from build123d import *

# Parameters (mm, degrees)
SKETCH_1_R      = 2.15
SKETCH_1_R_2    = 13.5
EXTRUDE_1_DEPTH = 5
FILLET_1_R      = 3
FILLET_2_R      = 1


with BuildPart() as part:
    # ｽｹｯﾁ1 → ﾎﾞｽ - 押し出し1 (new body)
    with BuildSketch(Plane(origin=(0, 0, 0), x_dir=(1, 0, 0), z_dir=(0, 1, 0))):
        with BuildLine():
            Line((-11.818899718, 2.076923077), (-16.328382426, -23.584655104))
            ThreePointArc((-16.328382426, -23.584655104), (-17.703637569, -26.24099819), (-20.349180229, -27.636917003))
            ThreePointArc((-20.349180229, -27.636917003), (-24.369978032, -31.689178902), (-21.971608059, -36.869474544))
            ThreePointArc((-21.971608059, -36.869474544), (-19.960473468, -39.083706455), (-19.573238085, -42.049770186))
            Line((-19.573238085, -42.049770186), (-20.683074506, -48.365384615))
            ThreePointArc((-20.683074506, -48.365384615), (-20.849535948, -54.509352655), (-19.230026487, -60.438369589))
            ThreePointArc((-19.230026487, -60.438369589), (-19.11671849, -64.1755701), (-21.627020352, -66.946470844))
            ThreePointArc((-21.627020352, -66.946470844), (-22.980970389, -74.980970389), (-14.946470844, -73.627020352))
            ThreePointArc((-14.946470844, -73.627020352), (-12.1755701, -71.11671849), (-8.438369589, -71.230026487))
            ThreePointArc((-8.438369589, -71.230026487), (-6.744432027, -71.887499507), (-5, -72.396078054))
            Line((-5, -72.396078054), (-5, -76.409830056))
            Line((-5, -76.409830056), (-2.666666667, -79.01857603))
            ThreePointArc((-2.666666667, -79.01857603), (3.651483717, -83.632993162), (-4, -82))
            Line((-4, -82), (-7.5, -82))
            ThreePointArc((-7.5, -82), (3.061862178, -88.846531969), (5, -76.409830056))
            Line((5, -76.409830056), (5, -72.396078054))
            ThreePointArc((5, -72.396078054), (6.744432027, -71.887499507), (8.438369589, -71.230026487))
            ThreePointArc((8.438369589, -71.230026487), (12.1755701, -71.11671849), (14.946470844, -73.627020352))
            ThreePointArc((14.946470844, -73.627020352), (22.980970389, -74.980970389), (21.627020352, -66.946470844))
            ThreePointArc((21.627020352, -66.946470844), (19.11671849, -64.1755701), (19.230026487, -60.438369589))
            ThreePointArc((19.230026487, -60.438369589), (20.849535948, -54.509352655), (20.683074506, -48.365384615))
            Line((20.683074506, -48.365384615), (19.573238085, -42.049770186))
            ThreePointArc((19.573238085, -42.049770186), (19.960473468, -39.083706455), (21.971608059, -36.869474544))
            ThreePointArc((21.971608059, -36.869474544), (24.369978032, -31.689178902), (20.349180229, -27.636917003))
            ThreePointArc((20.349180229, -27.636917003), (17.703637569, -26.24099819), (16.328382426, -23.584655104))
            Line((16.328382426, -23.584655104), (11.818899718, 2.076923077))
            ThreePointArc((11.818899718, 2.076923077), (0, 12), (-11.818899718, 2.076923077))
        make_face()
        with Locations(Location((-7.5, 0, 0), (0, 0, 270))):
            Circle(SKETCH_1_R, mode=Mode.SUBTRACT)
        with Locations(Location((7.5, 0, 0), (0, 0, 90))):
            Circle(SKETCH_1_R, mode=Mode.SUBTRACT)
        with Locations(Location((0, -52, 0), (0, 0, 270))):
            Circle(SKETCH_1_R_2, mode=Mode.SUBTRACT)
        with Locations(Location((19.445436483, -32.554563517, 0), (0, 0, 270))):
            Circle(SKETCH_1_R, mode=Mode.SUBTRACT)
        with Locations(Location((19.445436483, -71.445436483, 0), (0, 0, 270))):
            Circle(SKETCH_1_R, mode=Mode.SUBTRACT)
        with Locations(Location((-19.445436483, -71.445436483, 0), (0, 0, 270))):
            Circle(SKETCH_1_R, mode=Mode.SUBTRACT)
        with Locations(Location((-19.445436483, -32.554563517, 0), (0, 0, 270))):
            Circle(SKETCH_1_R, mode=Mode.SUBTRACT)
        with BuildLine():
            ThreePointArc((-4.384616486, -24.866395764), (0, -25.25), (4.384616486, -24.866395764))
            ThreePointArc((4.384616486, -24.866395764), (7.223675, -20.811800006), (3.169079242, -17.972741492))
            ThreePointArc((3.169079242, -17.972741492), (0, -18.25), (-3.169079242, -17.972741492))
            ThreePointArc((-3.169079242, -17.972741492), (-7.223675, -20.811800006), (-4.384616486, -24.866395764))
        make_face(mode=Mode.SUBTRACT)
    extrude(amount=EXTRUDE_1_DEPTH)

    # ﾌｨﾚｯﾄ1
    fillet_1_edges = [part.edges().sort_by_distance(p)[0] for p in [
        (5, 2.5, 72.396078054),
        (5, 2.5, 76.409830056),
        (-4, 2.5, 82),
        (-2.666666667, 2.5, 79.01857603),
        (-5, 2.5, 76.409830056),
        (-5, 2.5, 72.396078054),
    ]]
    fillet(fillet_1_edges, radius=FILLET_1_R)

    # ﾌｨﾚｯﾄ2
    fillet_2_edges = [part.edges().sort_by_distance(p)[0] for p in [
        (-7.5, 2.5, 82),
    ]]
    fillet(fillet_2_edges, radius=FILLET_2_R)


solid = part.part
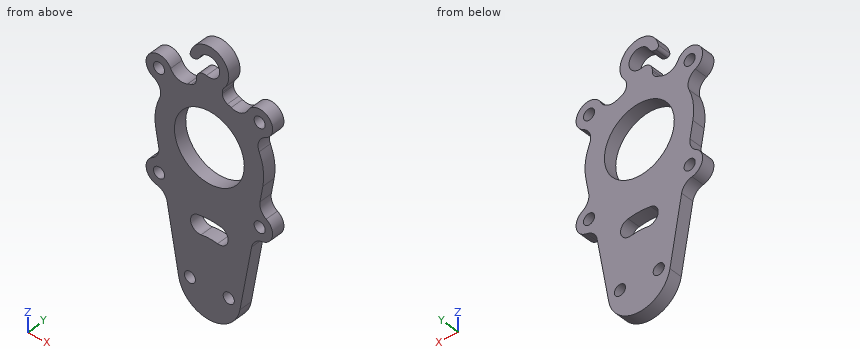
For this review, take the finished solid that the model builds, in its own axes (mm). Coordinates: 2 decimals unless noted, no trailing zeros. Loops run counter-clockwise (first coordinate to the right, second up) from the corner with the lowest first, then second, coordinate; pieces in that order, holes last. Notation, with made-up numbers: (3.25, 64) - (11.25, 64) arc R18 cw to (11.25, 77) - close; hole circle Ø3 at (58, 81.5). An arc over 180 degrees is marked (long way). Use a Markdown table: item, result. Add a question column.
Item 1: We need section C-C (z = 52). Give the boundary of the cut face in (x, y).
Item 2: Insertion check: pin 1 Ø2 at (y, z) = (3, 60.5) entering from +X; pin 2 Ø4 at (x, z) = (-19.45, 71.45) entering from +Y; pin 3 Ø13 at (x, z) = (0, 82) entering from +Y; pin 4 Ø1.5 at (y, z) = (4, 6) entering from +X. Each pin has a flat end and moves straight along its axis. Give the tip position at first contact, or say it passes through.
Item 3: We need section A-A (x = 0). Give the boundary of the cut face in (y, z), and give its area (4 significant figures).
Item 4: We need section D-D (y = 3.7). Give the number of separate pieces and of enclosed holes in the cut face, and give its area (3 significant figures).
Item 5: For line 1 (Z direction, x = -18.5, y = 1.7); line 2 (X direction, y = 3.1, z = 1.5); line 3 (Z direction, x = -0.5, y = 1.75), list the stretches that pass through material, from the lowest coordinate up.
Item 6: We need section B-B (z = -1). Give the boundary of the cut face in (x, y), and give its area (3 significant figures).
Results list:
| question | item | result |
|---|---|---|
| 1 | outline | (-21, 0) - (-13.5, 0) - (-13.5, 5) - (-21, 5) - close; (13.5, 0) - (21, 0) - (21, 5) - (13.5, 5) - close |
| 2 | pin 1 | stops at x = 19.62 |
| 2 | pin 2 | passes through |
| 2 | pin 3 | stops at y = 5 |
| 2 | pin 4 | stops at x = 13.37 |
| 3 | outline | (0, -12) - (5, -12) - (5, 18.25) - (0, 18.25) - close; (0, 25.25) - (5, 25.25) - (5, 38.5) - (0, 38.5) - close; (0, 65.5) - (5, 65.5) - (5, 78) - (0, 78) - close; (0, 86) - (5, 86) - (5, 89.5) - (0, 89.5) - close |
| 3 | area | 297.5 mm^2 |
| 4 | separate pieces | 1 |
| 4 | enclosed holes | 8 |
| 4 | area | 2,370 mm^2 |
| 5 | line 1 | z = 26.89 to 30.62, 34.49 to 69.51, 73.38 to 76.36 |
| 5 | line 2 | x = -12.45 to -9.04, -5.96 to 5.96, 9.04 to 12.45 |
| 5 | line 3 | z = -11.99 to 18.24, 25.25 to 38.51, 65.49 to 78.03, 85.97 to 89.48 |
| 6 | outline | (-12.01, 0) - (-9.4, 0) - (-9.4, 5) - (-12.01, 5) - close; (-5.6, 0) - (5.6, 0) - (5.6, 5) - (-5.6, 5) - close; (9.4, 0) - (12.01, 0) - (12.01, 5) - (9.4, 5) - close |
| 6 | area | 82.0 mm^2 |
